The model under review builds one solid part; all positions refer to its coordinate system, in mm. A direction names the side the tool comes from. Coordinates: 2 decimals unless noted, no trailing zeros. Loops run counter-clockwise (first coordinate to the right, second up) from the corner with the lowest first, then second, coordinate; pieces in that order, holes last. Notation, with made-up numbers: (62.25, 86.25) - (115.25, 86.25) arc R22 ccw to (115.25, 110.25) - close; hole circle Ø10 at (21, 49). An arc over 180 degrees is marked (long way). Answer in a Markdown table with one row per item. Add a question column.
(1) We need section D-D on x = 52.5. Write out the cut boundary in (y, z), plus the area to 3 significant figures.
(2) We need section C-C on z = 7. Write out the cut boundary in (x, y).
(3) Machinability: for faces 4 (the flat face through (77, 6, 7)), 5 (the flat face through (59.58, 1, 19)), 6 (the flat face through (55, 6, 20)), which of the approach directions +Z, -Z, +X, -X, +Y, -Y give a long, thin tool a straight path to every point of the face, cutting with its end or side? Answer none if there is none.
(4) We need section B-B on y = 1.5. Write out the cut boundary in (x, z), plus the area to 3 significant figures.
(5) For line 1 along Z through (x, y) = (63.5, 7.5); line 2 along Z through (x, y) = (35, 0.8); line 3 along X through (y, z) = (10, 5), list the stretches that pass through material, from the lowest coordinate up.
(6) Mouldability with a two-part tool opening along X and no side actions: class faces 1 (the flat face through (29, 6, 7)), 2 (the cylindrical face through (54.83, 14.43, 19.4)), 3 (the flat face through (54, 12, 7)) as +X half, -X half, draft (parallel to the pull), parting line (faces both ways), or undercut.
(7) For P1, Ø3, axis at x = 35.5, z = -8, coming from the +Y side; P2, Ø2.5, axis at x = 56.5, z = 18.5, coming from the -Y side; P3, Ø2.5, axis at y = 1, z = -8, coming from the +X side, all flat-tipped, find the tip position at first contact; note any pin that passes through.
(8) We need section A-A on x = 66. Write out the cut boundary in (y, z), plus the area to 3 significant figures.
Autodesk Inventor part; units mm, degrees
ref_plane "YZ Plane" through (0, 0, 0) normal (1, 0, 0) x (0, 1, 0)
ref_plane "XZ Plane" through (0, 0, 0) normal (0, 1, 0) x (-1, 0, 0)
ref_plane "XY Plane" through (0, 0, 0) normal (0, 0, 1) x (1, 0, 0)
sketch "Sketch1" plane through (0, 0, 0) normal (0, 1, 0) x (-1, 0, 0)
  line L0 (-77, 17) -> (-32, 17)
  line L1 (-32, 17) -> (-32, -3)
  line L2 (-32, -3) -> (-77, -3)
  line L3 (-77, -3) -> (-77, 17)
  line L4 (-78, 20) -> (-31, 20)
  line L5 (-29, 18) -> (-29, -4)
  line L6 (-41, -6) -> (-68, -6)
  line L7 (-80, -4) -> (-80, 18)
  arc A0 (-78, 20) -> (-80, 18) centre (-78, 18) ccw
  arc A1 (-29, 18) -> (-31, 20) centre (-31, 18) ccw
  arc A2 (-31, -6) -> (-29, -4) centre (-31, -4) ccw
  arc A3 (-80, -4) -> (-78, -6) centre (-78, -4) ccw
  line L8 (-77, -3) -> (-75.5, -3)
  line L9 (-75.5, -3) -> (-75.5, -1.5)
  circle A4 centre (-75.5, -1.5) radius 1
  line L10 (-32, 17) -> (-33.5, 17)
  line L11 (-33.5, 17) -> (-33.5, 15.5)
  circle A5 centre (-33.5, 15.5) radius 1
  line L12 (-49.42, 17) -> (-59.58, 17)
  line L13 (-59.58, 17) -> (-59.58, 14.46)
  line L14 (-59.58, 14.46) -> (-49.42, 14.46)
  line L15 (-49.42, 14.46) -> (-49.42, 17)
  line L16 (-78, -6) -> (-31, -6)
  line L17 (-77, -6) -> (-71, -6)
  line L18 (-71, -9) -> (-71, -9)
  line L19 (-74, -12) -> (-74, -12)
  line L20 (-77, -9) -> (-77, -6)
  line L21 (-32, -6) -> (-38, -6)
  line L22 (-38, -9) -> (-38, -9)
  line L23 (-35, -12) -> (-35, -12)
  line L24 (-32, -9) -> (-32, -6)
  arc A6 (-77, -9) -> (-74, -12) centre (-74, -9) ccw
  arc A7 (-74, -12) -> (-71, -9) centre (-74, -9) ccw
  arc A8 (-68, -6) -> (-71, -9) centre (-68, -9) ccw
  arc A9 (-38, -9) -> (-41, -6) centre (-41, -9) ccw
  arc A10 (-38, -9) -> (-35, -12) centre (-35, -9) ccw
  arc A11 (-35, -12) -> (-32, -9) centre (-35, -9) ccw
  circle A12 centre (-74, -9) radius 1.5
  circle A13 centre (-35, -9) radius 1.5
  line L25 (-77, -6) -> (-68, -6)
  line L26 (-41, -6) -> (-32, -6)
  point P0 (0, 0)
  point P1 (-38, -12)
  dimension "d44" = 45
  dimension "d45" = 20
  dimension "d46" = 2
  dimension "d47" = 1.5
  dimension "d48" = 1.5
  dimension "d49" = 2
  dimension "d50" = 1.5
  dimension "d51" = 1.5
  dimension "d52" = 2
  dimension "d53" = 10.16
  dimension "d54" = 2.54
  dimension "d55" = 3
  dimension "d56" = 3
  dimension "d57" = 3
extrude "Extrusion1" add sketch "Sketch1" along normal blind 3 contours L4 A1 L5 A2 L16 L6 A3 L7 A0 | L16 A8 A7 A6 L20 | L24 A11 A10 A9 L16
sketch "Sketch2" plane through (0, 3, 0) normal (0, 1, 0) x (1, 0, 0)
  line L0 (32, 3) -> (77, 3)
  line L1 (77, -17) -> (32, -17)
  line L2 (32, 3) -> (77, 3)
  line L3 (77, 3) -> (77, -17)
  line L4 (77, -17) -> (32, -17)
  line L5 (32, -17) -> (32, 3)
  line L6 (31, 6) -> (78, 6)
  line L7 (80, 4) -> (80, -18)
  line L8 (78, -20) -> (31, -20)
  line L9 (29, -18) -> (29, 4)
  arc A0 (31, 6) -> (29, 4) centre (31, 4) ccw
  arc A1 (80, 4) -> (78, 6) centre (78, 4) ccw
  arc A2 (78, -20) -> (80, -18) centre (78, -18) ccw
  arc A3 (29, -18) -> (31, -20) centre (31, -18) ccw
  point P0 (0, 0)
  dimension "d60" = 2
extrude "Extrusion2" add sketch "Sketch2" along normal blind 9
sketch "Sketch3" plane through (0, 12, 0) normal (0, 1, 0) x (1, 0, 0)
  line L0 (31, 6) -> (78, 6)
  line L1 (80, 4) -> (80, -18)
  line L2 (78, -20) -> (31, -20)
  line L3 (29, -18) -> (29, 4)
  arc A0 (31, 6) -> (29, 4) centre (31, 4) ccw
  arc A1 (80, 4) -> (78, 6) centre (78, 4) ccw
  arc A2 (78, -20) -> (80, -18) centre (78, -18) ccw
  arc A3 (29, -18) -> (31, -20) centre (31, -18) ccw
  point P0 (0, 0)
  dimension "d63" = 2
extrude "Extrusion3" add sketch "Sketch3" along normal blind 3
fillet "Fillet1" radius 2 8 edges at (29.5858, 15, -5.4142) (29, 15, 7) (29.5858, 15, 19.4142) (54.5, 15, 20) (79.4142, 15, 19.4142) (80, 15, 7) (79.4142, 15, -5.4142) (54.5, 15, -6)
sketch "Sketch4" plane through (0, 0, 0) normal (0, -1, 0) x (1, 0, 0)
  line L0 (31, 20) -> (78, 20)
  line L1 (54.5, 20) -> (49.42, 20)
  line L2 (49.42, 20) -> (59.58, 20)
  line L3 (59.58, 20) -> (59.58, 17)
  line L4 (77, 17) -> (32, 17)
  line L5 (49.42, 20) -> (49.42, 17)
  line L6 (49.42, 17) -> (59.58, 17)
  point P0 (0, 0)
  dimension "d67" = 5.08
  dimension "d68" = 10.16
extrude "Extrusion4" cut sketch "Sketch4" against normal blind 2.54
sketch "Sketch5" plane through (0, 15, 0) normal (0, 1, 0) x (1, 0, 0)
  line L0 (78, -18) -> (31, -18)
  line L1 (31, 4) -> (78, 4)
  circle A0 centre (43, -7) radius 9
  circle A1 centre (66, -7) radius 9
  point P0 (0, 0)
extrude "Extrusion5" cut sketch "Sketch5" against normal blind 3
Outcome:
| question | item | result |
|---|---|---|
| 1 | outline | (0, -6) - (13, -6) arc R2 ccw to (15, -4) - (15, 18) arc R2 ccw to (13, 20) - (2.54, 20) - (2.54, 17) - (12, 17) - (12, -3) - (0, -3) - close |
| 1 | area | 141 mm² |
| 2 | outline | (29, 0) - (32, 0) - (32, 12) - (34, 12) - (34, 15) - (31, 15) arc R2 ccw to (29, 13) - close; (52, 12) - (57, 12) - (57, 15) - (52, 15) - close; (75, 12) - (77, 12) - (77, 0) - (80, 0) - (80, 13) arc R2 ccw to (78, 15) - (75, 15) - close |
| 3 | face 4 | -Y |
| 3 | face 5 | +Z, -Y |
| 3 | face 6 | +Z, +X, -X, +Y, -Y |
| 4 | outline | (29, -4) arc R2 ccw to (31, -6) - (32, -6) - (32, -9) arc R3 ccw to (38, -9) arc R3 cw to (41, -6) - (68, -6) arc R3 cw to (71, -9) arc R3 ccw to (77, -9) - (77, -6) - (78, -6) arc R2 ccw to (80, -4) - (80, 18) arc R2 ccw to (78, 20) - (59.58, 20) - (59.58, 17) - (77, 17) - (77, -3) - (32, -3) - (32, 17) - (49.42, 17) - (49.42, 20) - (31, 20) arc R2 ccw to (29, 18) - close; hole circle Ø3 at (35, -9); hole circle Ø3 at (74, -9) |
| 4 | area | 446 mm² |
| 5 | line 1 | -6 to -3, 17 to 20 |
| 5 | line 2 | -12 to -10.5, -7.5 to -3, 17 to 20 |
| 5 | line 3 | 29 to 32, 77 to 80 |
| 6 | face 1 | -X half |
| 6 | face 2 | draft |
| 6 | face 3 | undercut |
| 7 | P1 | y = 3 |
| 7 | P2 | y = 2.54 |
| 7 | P3 | x = 77 |
| 8 | outline | (0, -6) - (13, -6) arc R2 ccw to (15, -4) - (15, -2) - (12, -2) - (12, -3) - (0, -3) - close; (0, 17) - (12, 17) - (12, 16) - (15, 16) - (15, 18) arc R2 ccw to (13, 20) - (0, 20) - close |
| 8 | area | 94.3 mm² |
